Can you work these out from the model? Positions are in its coordinate system, mm. Face numbers are marked on the shaded views. A direction names the side the tool comes from. Round coordinates to 2 decimals unless told otherwise and drop trailing zeros. Order: outer loops, then holes, each group sorted by start corner. A loop starts at its lowest first (then second) coordinate and runs counter-clockwise, first axis right, second up.
Autodesk Inventor part; units mm, degrees
ref_plane "Pracovní rovina1" through (12, -8, -9.8) normal (0, 0, 1) x (1, 0, 0)
ref_plane "YZ Plane" through (0, 0, 0) normal (1, 0, 0) x (0, 1, 0)
ref_plane "XZ Plane" through (0, 0, 0) normal (0, 1, 0) x (-1, 0, 0)
sketch "Náčrt1" plane through (0, 0, 0) normal (0, 0, 1) x (1, 0, 0)
  line L0 (0, 12.6) -> (0, -12.6)
  line L1 (-12.6, 0) -> (12.6, 0)
  line L2 (-9, 9) -> (9, 9)
  line L3 (9, 9) -> (9, -9)
  line L4 (9, -9) -> (-9, -9)
  line L5 (-9, -9) -> (-9, 9)
  point P0 (0, 0)
  dimension "d0" = 18
  dimension "d1" = 18
extrude "Vysunutí1" add sketch "Náčrt1" against normal blind 20
sketch "Náčrt2" plane through (-9, 9, 0) normal (0, 1, 0) x (1, 0, 0)
  line L0 (18, 0) -> (0, 0)
  line L1 (18, 0) -> (18, 20)
  line L2 (0, 20) -> (18, 20)
  line L3 (0, 0) -> (0, 20)
  line L4 (1.3, 16.6) -> (1.3, 3)
  line L5 (1.3, 3) -> (16.7, 3)
  line L6 (16.7, 3) -> (16.7, 16.6)
  line L7 (16.7, 16.6) -> (1.3, 16.6)
  point P0 (9, 0)
  dimension "d4" = 3.4
  dimension "d5" = 3
  dimension "d6" = 1.3
  dimension "d7" = 1.3
sketch "Náčrt3" plane through (0, 0, 0) normal (0, 0, 1) x (1, 0, 0)
  point P0 (0, 0)
extrude "Vysunutí2" cut sketch "Náčrt2" against normal blind 17 contours L7 L6 L5 L4
sketch "Náčrt4" plane through (0, 0, 0) normal (0, 0, 1) x (1, 0, 0)
  line L0 (0, 12.6) -> (0, -12.6)
  line L1 (-12.6, 0) -> (12.6, 0)
  circle A0 centre (0, -4) radius 3.1
  line L2 (-9, -9) -> (9, -9)
  point P0 (0, 0)
  dimension "d10" = 6.2
  dimension "d11" = 5
extrude "Vysunutí3" cut sketch "Náčrt4" against normal blind 3
sketch "Náčrt5" plane through (-9, 9, 0) normal (0, 1, 0) x (1, 0, 0)
  line L0 (1.3, 3) -> (1.3, 16.6)
  line L1 (1.3, 16.6) -> (16.7, 16.6)
  line L2 (16.7, 3) -> (1.3, 3)
  line L3 (16.7, 16.6) -> (16.7, 3)
  line L4 (1.3, 16.6) -> (16.7, 16.6)
  line L5 (1.3, 3) -> (1.3, 16.6)
  line L6 (16.7, 16.6) -> (16.7, 3)
  line L7 (16.7, 16.6) -> (16.7, 3)
  line L8 (16.7, 3) -> (1.3, 3)
  line L9 (1.3, 3) -> (1.3, 16.6)
  line L10 (1.3, 16.6) -> (16.7, 16.6)
  line L11 (18, 0) -> (0, 0)
  line L12 (18, 0) -> (18, 20)
  line L13 (0, 20) -> (18, 20)
  line L14 (0, 0) -> (0, 20)
  line L15 (1.3, 16.6) -> (0, 16.6)
  line L16 (0, 0) -> (0, 20)
  line L17 (0, 16.6) -> (0, 0)
  line L18 (0, 0) -> (18, 0)
  line L19 (18, 0) -> (18, 16.6)
  line L20 (18, 0) -> (18, 20)
  line L21 (16.7, 16.6) -> (18, 16.6)
  line L22 (16.7, 16.6) -> (16.7, 3)
  line L23 (16.7, 3) -> (1.3, 3)
  line L24 (16.7, 3) -> (1.3, 3)
  line L25 (1.3, 3) -> (1.3, 16.6)
  line L26 (1.3, 3) -> (1.3, 16.6)
  point P0 (9, 0)
extrude "Vysunutí4" cut sketch "Náčrt5" against normal blind 8 contours L2 L3 L21 L12 L11 L14 L15 L0
sketch "Náčrt6" plane through (0, 0, -20) normal (0, 0, -1) x (-1, 0, 0)
  line L0 (-9, -9) -> (9, -9)
  line L1 (9, -9) -> (9, 9)
  line L2 (9, 9) -> (-9, 9)
  line L3 (-9, 9) -> (-9, -9)
  line L4 (0, -12.6) -> (0, 12.6)
  line L5 (-12.6, 0) -> (12.6, 0)
  line L6 (-2.8665, 6.0827) -> (2.9335, 6.0827)
  line L7 (2.9335, 6.0827) -> (2.9335, -5.9173)
  line L8 (2.9335, -5.9173) -> (-2.8665, -5.9173)
  line L9 (-2.8665, -5.9173) -> (-2.8665, 6.0827)
  point P0 (0, 0)
  dimension "d16" = 5.8
  dimension "d17" = 12
extrude "Vysunutí5" cut sketch "Náčrt6" against normal blind 8 contours L8 L9 L5 L4 | L4 L5 L7 L8 | L9 L6 L4 L5 | L4 L6 L7 L5
sketch "Náčrt13" plane through (9, -9, -20) normal (1, 0, 0) x (0, 0, -1)
  line L0 (-3.4, 10) -> (-20, 10)
  line L1 (-20, 0) -> (-20, 10)
  line L2 (-20, 0) -> (0, 0)
  line L3 (0, 18) -> (0, 0)
  line L4 (-3.4, 18) -> (0, 18)
  line L5 (-3.4, 18) -> (-3.4, 10)
  line L6 (-3.4, 1) -> (-17, 1)
  line L7 (-17, 1) -> (-3.4, 1)
  line L8 (-17, 10) -> (-3.4, 10)
  line L9 (-17, 1) -> (-17, 10)
  line L10 (-17, 8.1) -> (-17, 1.9)
  line L11 (-3.4, 1) -> (-3.4, 10)
  line L12 (-3.4, 1) -> (-17, 1)
  line L13 (-3.4, 10) -> (-17, 10)
  point P0 (-20, 9)
extrude "Vysunutí11" cut sketch "Náčrt13" against normal blind 20 contours L11 L6 L9 L0
sketch "Náčrt14" plane through (0, 0, 0) normal (0, 0, 1) x (1, 0, 0)
  line L0 (9, 1) -> (-9, 1)
  line L1 (-9, 1) -> (-9, -9)
  line L2 (-9, -9) -> (9, -9)
  line L3 (9, -9) -> (9, 1)
  circle A0 centre (0, -4) radius 3.1
  line L4 (2.8665, -5.9173) -> (-2.9335, -5.9173)
  line L5 (9, -8) -> (-9, -8)
  line L6 (9, -8) -> (-9, -8)
  line L7 (9, 1) -> (6.5, 1)
  line L8 (6.5, 1) -> (6.5, -8)
  line L9 (6.5, -8) -> (9, -8)
  line L10 (9, -8) -> (9, 1)
  line L11 (-9, 1) -> (-6.5, 1)
  line L12 (-6.5, 1) -> (-6.5, -8)
  line L13 (-6.5, -8) -> (-9, -8)
  line L14 (-9, -8) -> (-9, 1)
  point P0 (0, 0)
  dimension "d44" = 2.5
  dimension "d45" = 2.5
extrude "Vysunutí12" cut sketch "Náčrt14" against normal blind 5 contours L3 L5 L8 L0 | L12 L5 L1 L0
sketch "Náčrt15" plane through (-9, -9, 0) normal (0, -1, 0) x (1, 0, 0)
  line L0 (0, 0) -> (18, 0)
  line L1 (0, 0) -> (0, -20)
  line L2 (18, -20) -> (0, -20)
  line L3 (18, 0) -> (18, -20)
  line L4 (18, 0) -> (0, 0)
  line L5 (0, 0) -> (0, -20)
  line L6 (0, -20) -> (18, -20)
  line L7 (18, -20) -> (18, 0)
  point P0 (9, 0)
extrude "Vysunutí13" add sketch "Náčrt15" along normal blind 1.2
sketch "Náčrt16" plane through (9, -8, -16.6) normal (1, 0, 0) x (0, 0, -1)
  line L0 (0, 0) -> (-16.6, 0)
  line L1 (-16.6, -2.2) -> (-16.6, 0)
  line L2 (3.4, -2.2) -> (-16.6, -2.2)
  line L3 (3.4, 17) -> (3.4, -2.2)
  line L4 (0, 17) -> (3.4, 17)
  line L5 (0, 17) -> (0, 0)
  line L6 (-16.6, 0) -> (3.4, 0)
  line L7 (3.4, 0) -> (3.4, -2.2)
  line L8 (3.4, -2.2) -> (-16.6, -2.2)
  line L9 (-16.6, -2.2) -> (-16.6, 0)
  line L10 (0, 17) -> (3.4, 17)
  line L11 (3.4, 17) -> (3.4, 0)
  line L12 (3.4, 0) -> (0, 0)
  line L13 (0, 0) -> (0, 17)
  point P0 (-16.6, 8)
extrude "Vysunutí14" add sketch "Náčrt16" along normal blind 3
sketch "Náčrt17" plane through (-9, -8, -16.6) normal (-1, 0, 0) x (0, 0, 1)
  line L0 (16.6, 0) -> (0, 0)
  line L1 (0, 0) -> (0, 17)
  line L2 (0, 17) -> (-3.4, 17)
  line L3 (-3.4, 17) -> (-3.4, -2.2)
  line L4 (16.6, -2.2) -> (-3.4, -2.2)
  line L5 (16.6, 0) -> (16.6, -2.2)
  line L6 (-3.4, 17) -> (0, 17)
  line L7 (0, 17) -> (0, -2.2)
  line L8 (0, -2.2) -> (-3.4, -2.2)
  line L9 (-3.4, -2.2) -> (-3.4, 17)
  line L10 (16.6, 0) -> (0, 0)
  line L11 (0, 0) -> (0, -2.2)
  line L12 (0, -2.2) -> (16.6, -2.2)
  line L13 (16.6, -2.2) -> (16.6, 0)
  point P0 (16.6, 8)
  point P1 (0, -1.1)
  dimension "d52" = 3.4
extrude "Vysunutí15" add sketch "Náčrt17" along normal blind 3
sketch "Náčrt18" plane through (0, 0, -20) normal (0, 0, -1) x (-1, 0, 0)
  line L0 (2.9335, 6.0827) -> (2.9335, -5.9173)
  line L1 (2.9335, -5.9173) -> (-2.8665, -5.9173)
  line L2 (-2.8665, -5.9173) -> (-2.8665, 6.0827)
  line L3 (-2.8665, 6.0827) -> (2.9335, 6.0827)
  line L4 (-12, 9) -> (12, 9)
  line L5 (-12, -10.2) -> (-12, 9)
  line L6 (-12, -10.2) -> (12, -10.2)
  line L7 (12, 9) -> (12, -10.2)
  line L8 (-12, 9) -> (12, 9)
  line L9 (12, 9) -> (12, -10.2)
  line L10 (12, -10.2) -> (-12, -10.2)
  line L11 (-12, -10.2) -> (-12, 9)
  line L12 (-2.8665, 6.0827) -> (2.9335, 6.0827)
  line L13 (2.9335, 6.0827) -> (2.9335, -5.9173)
  line L14 (2.9335, -5.9173) -> (-2.8665, -5.9173)
  line L15 (-2.8665, -5.9173) -> (-2.8665, 6.0827)
  point P0 (0, 0)
extrude "Vysunutí16" add sketch "Náčrt18" along normal blind 1.6
sketch "Náčrt19" plane through (12, -8, -16.6) normal (0, 0, 1) x (1, 0, 0)
  line L0 (-24, 17) -> (0, 17)
  line L1 (0, 0) -> (-24, 0)
  line L2 (-16.5, 17) -> (-7.5, 17)
  line L3 (-7.5, 17) -> (-7.5, 0)
  line L4 (-7.5, 0) -> (-16.5, 0)
  line L5 (-16.5, 0) -> (-16.5, 17)
  line L6 (-14.9335, 2.0827) -> (-14.9335, 14.0827)
  line L7 (-14.9335, 14.0827) -> (-9.1335, 14.0827)
  line L8 (-9.1335, 14.0827) -> (-9.1335, 2.0827)
  line L9 (-9.1335, 2.0827) -> (-14.9335, 2.0827)
  line L10 (0, 0) -> (-24, 0)
  line L11 (0, 17) -> (0, 0)
  line L12 (-24, 17) -> (0, 17)
  line L13 (-24, 0) -> (-24, 17)
  line L14 (-12, 17) -> (-12, 0)
  line L15 (-16.5, 17) -> (-7.5, 17)
  line L16 (-16.5, 0) -> (-7.5, 0)
  point P0 (-12, 8)
  point P1 (-16.5, 0)
  dimension "d57" = 9
ref_plane "Pracovní rovina1" through (12, -8, -9.8) normal (0, 0, 1) x (1, 0, 0)
extrude "Vysunutí17" cut sketch "Náčrt19" against normal blind 3 contours L0 L14 L7 L6 L9 L1 L5 | L0 L3 L1 L14 L9 L8 L7
sketch "Náčrt20" plane through (-12, 9, -21.6) normal (0, 1, 0) x (1, 0, 0)
  line L0 (0, -5) -> (0, 0)
  line L1 (24, -5) -> (24, 0)
  line L2 (0, 0) -> (24, 0)
  line L3 (24, 0) -> (24, -5)
  line L4 (24, -5) -> (0, -5)
  line L5 (0, -5) -> (0, 0)
  point P0 (12, -21.6)
extrude "Vysunutí18" add sketch "Náčrt20" along normal blind 4
sketch "Náčrt21" plane through (4.5, -8, -16.6) normal (0, 0, 1) x (1, 0, 0)
  line L0 (0, 17) -> (0, 0)
  line L1 (7.5, 0) -> (0, 0)
  line L2 (7.5, 0) -> (7.5, 21)
  line L3 (-16.5, 21) -> (7.5, 21)
  line L4 (-16.5, 0) -> (-16.5, 21)
  line L5 (-9, 0) -> (-16.5, 0)
  line L6 (-9, 0) -> (-9, 17)
  line L7 (-9, 17) -> (0, 17)
  circle A0 centre (-11.5, 18) radius 0.95
  circle A1 centre (2.5, 3) radius 0.95
  line L8 (7.5, 10.5) -> (-16.5, 10.5)
  circle A2 centre (2.5, 18) radius 0.95
  circle A3 centre (-11.5, 3) radius 0.95
  point P0 (-4.5, 8)
  dimension "d62" = 1.9
  dimension "d63" = 3
  dimension "d64" = 5
  dimension "d65" = 1.9
  dimension "d66" = 3
  dimension "d67" = 5
extrude "Vysunutí19" cut sketch "Náčrt21" against normal up to surface (5 mm away) contours A0 | A1 | A2 | A3
sketch "Náčrt22" plane through (-12, 13, -21.6) normal (0, 1, 0) x (1, 0, 0)
  line L0 (0, 0) -> (0, -5)
  line L1 (0, -5) -> (24, -5)
  line L2 (24, -5) -> (24, 0)
  line L3 (24, 0) -> (0, 0)
  line L4 (5.5, -21.6) -> (0, -21.6)
  line L5 (5.5, -21.6) -> (5.5, -18.6)
  line L6 (18.5, -18.6) -> (5.5, -18.6)
  line L7 (18.5, -21.6) -> (18.5, -18.6)
  line L8 (18.5, -21.6) -> (24, -21.6)
  line L9 (24, -5) -> (24, -21.6)
  line L10 (24, -5) -> (16.5, -5)
  line L11 (16.5, -5) -> (16.5, -2)
  line L12 (16.5, -2) -> (7.5, -2)
  line L13 (7.5, -5) -> (7.5, -2)
  line L14 (7.5, -5) -> (0, -5)
  line L15 (0, -21.6) -> (0, -5)
  line L16 (5.5, -18.6) -> (5.5, -21.6)
  line L17 (18.5, -21.6) -> (5.5, -21.6)
  line L18 (18.5, -21.6) -> (18.5, -18.6)
  line L19 (18.5, -18.6) -> (5.5, -18.6)
  line L20 (24, 0) -> (22, 0)
  line L21 (22, 0) -> (22, -21.6)
  line L22 (22, -21.6) -> (24, -21.6)
  line L23 (24, -21.6) -> (24, 0)
  line L24 (0, 0) -> (2, 0)
  line L25 (2, 0) -> (2, -21.6)
  line L26 (2, -21.6) -> (0, -21.6)
  line L27 (0, -21.6) -> (0, 0)
  point P0 (12, -21.6)
  dimension "d71" = 2
  dimension "d72" = 2
extrude "Vysunutí20" cut sketch "Náčrt22" against normal through all contours L3 L25 L1 L0 | L1 L25 L4 L15 | L3 L2 L1 L21 | L1 L9 L8 L21
sketch "Náčrt23" plane through (0, 0, 0) normal (0, 0, 1) x (1, 0, 0)
  line L0 (10, -10.2) -> (10, -8)
  line L1 (6.5, -8) -> (10, -8)
  line L2 (6.5, -8) -> (6.5, 1)
  line L3 (6.5, 1) -> (-6.5, 1)
  line L4 (-6.5, 1) -> (-6.5, -8)
  line L5 (-6.5, -8) -> (-10, -8)
  line L6 (-10, -8) -> (-10, -10.2)
  line L7 (-10, -10.2) -> (10, -10.2)
  circle A0 centre (0, -4) radius 3.1
  line L8 (-10, -8) -> (10, -8)
  line L9 (10, -8) -> (10, -10.2)
  line L10 (10, -10.2) -> (-10, -10.2)
  line L11 (-10, -10.2) -> (-10, -8)
  point P0 (0, 0)
extrude "Vysunutí21" add sketch "Náčrt23" along normal blind 4 contours L7 L6 L5 L8 L1 L0
sketch "Náčrt24" plane through (-9, -8, 0) normal (0, 1, 0) x (1, 0, 0)
  line L0 (2.5, 3) -> (2.5, 0)
  line L1 (15.5, 0) -> (2.5, 0)
  line L2 (15.5, 0) -> (15.5, 3)
  line L3 (15.5, 3) -> (2.5, 3)
  line L4 (2.5, 0) -> (2.5, 3)
  line L5 (15.5, 3) -> (2.5, 3)
  line L6 (15.5, 0) -> (15.5, 3)
  line L7 (2.5, 0) -> (15.5, 0)
  line L8 (-1, 16.6) -> (-1, -4)
  line L9 (19, -4) -> (-1, -4)
  line L10 (19, -4) -> (19, 16.6)
  line L11 (19, 16.6) -> (13.5, 16.6)
  line L12 (13.5, 16.6) -> (13.5, 19.6)
  line L13 (13.5, 19.6) -> (4.5, 19.6)
  line L14 (4.5, 16.6) -> (4.5, 19.6)
  line L15 (4.5, 16.6) -> (-1, 16.6)
  line L16 (15.5, 3) -> (2.5, 3)
  line L17 (2.5, 3) -> (2.5, 0)
  line L18 (2.5, -1) -> (15.5, -1)
  line L19 (15.5, -1) -> (15.5, -4)
  line L20 (15.5, -4) -> (2.5, -4)
  line L21 (2.5, -4) -> (2.5, -1)
  line L22 (11.8665, 21.6) -> (6.0665, 21.6)
  point P0 (9, 0)
  point P1 (15.5, -2.5)
  point P2 (2.5, -4)
  dimension "d77" = 3
  dimension "d78" = 13
  dimension "d87" = 3.5
extrude "Vysunutí22" add sketch "Náčrt24" along normal up to surface (9 mm away) contours L21 L18 L19 L9
sketch "Náčrt25" plane through (0, 0, 4) normal (0, 0, 1) x (1, 0, 0)
  line L0 (10, -8) -> (6.5, -8)
  line L1 (6.5, -8) -> (6.5, 1)
  line L2 (-6.5, 1) -> (6.5, 1)
  line L3 (-6.5, -8) -> (-6.5, 1)
  line L4 (-6.5, -8) -> (-10, -8)
  line L5 (-10, -8) -> (-10, -10.2)
  line L6 (-10, -10.2) -> (10, -10.2)
  line L7 (10, -10.2) -> (10, -8)
  circle A0 centre (0, -4) radius 3.1
  circle A1 centre (0, -4) radius 3.1
  point P0 (0, 0)
extrude "Vysunutí23" cut sketch "Náčrt25" against normal blind 10 contours A0
sketch "Náčrt26" plane through (-9, 1, 0) normal (0, 1, 0) x (1, 0, 0)
  line L0 (2.5, 3) -> (2.5, 0)
  line L1 (15.5, 0) -> (2.5, 0)
  line L2 (15.5, 0) -> (15.5, 3)
  line L3 (15.5, 3) -> (2.5, 3)
  line L4 (2.5, 3) -> (15.5, 3)
  line L5 (15.5, 3) -> (15.5, 0)
  line L6 (15.5, 0) -> (2.5, 0)
  line L7 (2.5, 0) -> (2.5, 3)
  line L8 (2.5, 3) -> (15.5, 3)
  line L9 (15.5, 3) -> (15.5, 0)
  line L10 (15.5, 0) -> (2.5, 0)
  line L11 (2.5, 0) -> (2.5, 3)
  point P0 (9, 0)
extrude "Vysunutí24" cut sketch "Náčrt26" against normal up to surface (9 mm away)
properties part number "laser_krabicka2_3D tisk"
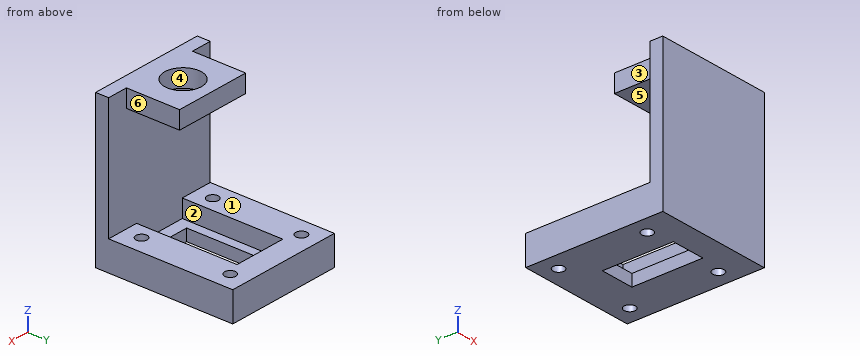
(1) On a 3-axis mill with a long thin cutter (end or side, diameter ignored), from which of +Z, -Z, +X, -X, +Y, -Y can I reach the whole of each face in a straight line? I mean the marked faces 4, 5 and 6. Say none if no direction works.
(2) I want a section at A-A, the plane y = 10. List the corners of the cut face in (x, z) for me.
(3) I want a section at D-D, the plane y = 2.25. List the corners of the cut face in (x, z) for me.
(4) Please list where these lines run through material, in increasing order: probe 1 along Y at (x, z) = (-7, -17.6); probe 2 along Z at (x, y) = (-4, -4.75); probe 3 along Z at (x, y) = (5.75, -5).
(5) If we mould it in two halves opening along X, with no side actions, what happens to the marked faces 1, 2 and 3? For each: pulls with the +X half, pulls with the -X half, needs draft (parallel to the pull), parting line crosses it, or undercut.
(6) I want a section at C-C, the plane z = -17.5. List the corners of the cut face in (x, y) for me.
(7) I want a section at B-B, the plane x = 0. List the corners of the cut face in (y, z) for me, plus the area to 3 significant figures.
(8) I'm going to push flat-ended pins straight in: pin 1 Ø1.7 at (x, y) = (-7, 10) entering from +Z; pin 2 Ø5 at (x, y) = (0, -4) entering from +Z; pin 3 Ø1.5 at (x, y) = (-7, -5) entering from -Z; pin 4 Ø1.5 at (x, z) = (1, -10.5) entering from +Y. Where does each tip first touch, or does it pass through?
Ans:
1. face 4: +Z
1. face 5: +X, -X, +Y
1. face 6: +Z, +X, +Y
2. outline: (-10, -21.6) - (-7.95, -21.6) - (-7.95, -16.6) - (-10, -16.6) - close; (-6.05, -21.6) - (6.05, -21.6) - (6.05, -16.6) - (-6.05, -16.6) - close; (7.95, -21.6) - (10, -21.6) - (10, -16.6) - (7.95, -16.6) - close
3. outline: (-10, -21.6) - (-2.93, -21.6) - (-2.93, -19.6) - (-4.5, -19.6) - (-4.5, -16.6) - (-10, -16.6) - close; (2.87, -21.6) - (10, -21.6) - (10, -16.6) - (4.5, -16.6) - (4.5, -19.6) - (2.87, -19.6) - close
4. probe 1: y = -10.2 to -5.95, -4.05 to 9.05, 10.95 to 13
4. probe 2: z = -21.6 to -19.6, 1 to 4
4. probe 3: z = -21.6 to -16.6, 1 to 4
5. face 1: needs draft
5. face 2: undercut
5. face 3: pulls with the -X half
6. outline: (-10, -10.2) - (10, -10.2) - (10, 13) - (-10, 13) - close; hole circle Ø1.9 at (-7, -5); hole circle Ø1.9 at (-7, 10); hole (-4.5, -8) - (4.5, -8) - (4.5, 9) - (-4.5, 9) - close; hole circle Ø1.9 at (7, -5); hole circle Ø1.9 at (7, 10)
7. outline: (-10.2, -21.6) - (-5.92, -21.6) - (-5.92, -19.6) - (-8, -19.6) - (-8, 1) - (-7.1, 1) - (-7.1, 4) - (-10.2, 4) - close; (-0.9, 1) - (1, 1) - (1, 4) - (-0.9, 4) - close; (6.08, -21.6) - (13, -21.6) - (13, -16.6) - (9, -16.6) - (9, -19.6) - (6.08, -19.6) - close
7. area: 94.7 mm2
8. pin 1: passes through
8. pin 2: stops at z = -19.6
8. pin 3: stops at z = 1
8. pin 4: stops at y = -8
